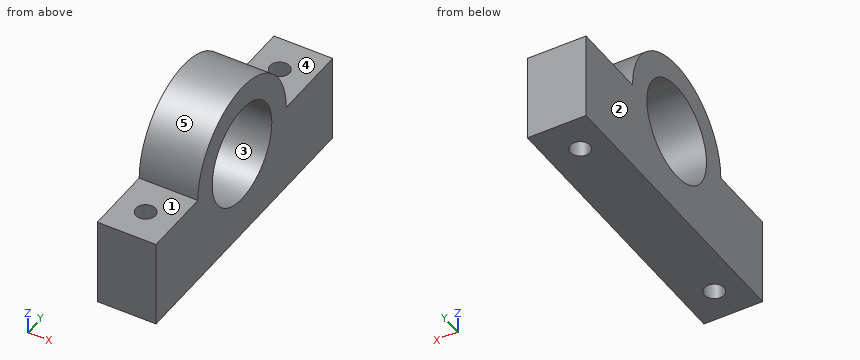
```python
from build123d import *

# Parameters (mm, degrees)
F1_DEPTH = 12.7
F2_R     = 2.1209
F3_DEPTH = 25.4
F4_R     = 2.1209
F5_DEPTH = 25.4


with BuildPart() as f1:
    # F0 (on Right) → F1 (new body)
    with BuildSketch(Plane.YZ):
        with BuildLine():
            Line((10.7188, 0), (15.875, 0))
            ThreePointArc((15.875, 0), (0, 15.875), (-15.875, 0))
            Line((-15.875, 0), (-10.7188, 0))
            ThreePointArc((-10.7188, 0), (0, 10.7188), (10.7188, 0))
        make_face()
        with BuildLine():
            Line((32.5907057375, 0), (15.875, 0))
            ThreePointArc((15.875, 0), (0, -15.875), (-15.875, 0))
            Line((-15.875, 0), (-30.9092942625, 0))
            Line((-30.9092942625, 0), (-30.9092942625, -19.05))
            Line((-30.9092942625, -19.05), (32.5907057375, -19.05))
            Line((32.5907057375, -19.05), (32.5907057375, 0))
        make_face()
        with BuildLine():
            ThreePointArc((-15.875, 0), (0, -15.875), (15.875, 0))
            Line((15.875, 0), (10.7188, 0))
            ThreePointArc((10.7188, 0), (0, -10.7188), (-10.7188, 0))
            Line((-10.7188, 0), (-15.875, 0))
        make_face()
    extrude(amount=F1_DEPTH)

    # F2 (on face) → F3 (cut)
    with BuildSketch(Plane.XY):
        with Locations((5.9564788826, 24.7918274254)):
            Circle(F2_R)
    extrude(amount=-F3_DEPTH, mode=Mode.SUBTRACT)

    # F4 (on face) → F5 (cut)
    with BuildSketch(Plane.XY):
        with Locations((6.1368788593, -23.7293746322)):
            Circle(F4_R)
    extrude(amount=-F5_DEPTH, mode=Mode.SUBTRACT)


solid = f1.part
```
Model file for the job. Use its own axes, mm. Face numbers are marked on the shaded views. A direction names the side the tool comes from. Coordinates: 2 decimals unless noted, no trailing zeros. Order: outer loops, then holes, each group sorted by start corner. A loop starts at its lowest first (then second) coordinate and runs counter-clockwise, first axis right, second up. Notation, with made-up numbers: (66, 54.5) -> (122, 54.5) arc R7 cw to (122, 63.5) -> close; hole circle Ø8 at (-37.75, 70). An arc over 180 degrees is marked (long way). Return JSON: item names as keys, results as strings.
Item 1: Slice it at D-D (x = 9.75). Write the cut outline in (y, z) (3 decimals), then the cut area to 3 significant figures.
Model answer:
{"outline": "(-30.909, -19.05) -> (32.591, -19.05) -> (32.591, 0) -> (15.875, 0) arc R15.875 ccw to (-15.875, 0) -> (-30.909, 0) -> close; hole circle Ø21.438 at (0, 0)", "area": "1,240 mm²"}
Item 2: Mould opens along Z. For the marked faces 1, 2 and 3 say: pulls with the +Z half, pulls with the -Z half, needs draft (parallel to the pull), parting line crosses it, or undercut.
Model answer:
{"face 1": "pulls with the +Z half", "face 2": "needs draft", "face 3": "undercut"}
Item 3: Slice it at A-A (y = 0). Write the cut outline in (x, z) (3 decimals).
Model answer:
{"outline": "(0, -19.05) -> (12.7, -19.05) -> (12.7, -10.719) -> (0, -10.719) -> close; (0, 10.719) -> (12.7, 10.719) -> (12.7, 15.875) -> (0, 15.875) -> close"}
Item 4: Slice it at B-B (z = -2). Write the cut outline in (x, y).
Model answer:
{"outline": "(0, -30.91) -> (12.7, -30.91) -> (12.7, -10.53) -> (0, -10.53) -> close; (0, 10.53) -> (12.7, 10.53) -> (12.7, 32.59) -> (0, 32.59) -> close; hole circle Ø4.24 at (5.96, 24.79); hole circle Ø4.24 at (6.14, -23.73)"}
Item 5: 3-axis set-ups, long thin cutter, end or side, ignore diameter. For the marked faces 4 and 5: which of +Z, -Z, +X, -X, +Y, -Y reach the whole face in a straight line?
Model answer:
{"face 4": "+Z, +X, -X, +Y", "face 5": "+Z, +X, -X"}
Item 6: Wall check: line 1 along Y through (x, z) = (7, -13.5); line 2 along Z through (x, y) = (7.75, 0) (3 decimals); line 3 along Y through (x, z) = (4.75, -3). Give the ranges that are in metal, low to high. Write a range as from..to.
Model answer:
{"line 1": "y = -30.91..-25.67, -21.79..22.95, 26.64..32.59", "line 2": "z = -19.05..-10.719, 10.719..15.875", "line 3": "y = -30.91..-25.33, -22.12..-10.29, 10.29..23.05, 26.54..32.59"}
Item 7: Pin check, flat tips, straight feed: P1, Ø5, axis at x = 6.14, y = -23.73, coming from the +Z side; P2, Ø5, axis at x = 3, z = 5, coming from the +Y side. Stop position of each tip, or through.
Model answer:
{"P1": "stops at z = 0", "P2": "stops at y = 15.68"}
Item 8: Slice it at C-C (x = 5.75). Write the cut outline in (y, z) (3 decimals).
Model answer:
{"outline": "(-30.909, -19.05) -> (-25.815, -19.05) -> (-25.815, 0) -> (-30.909, 0) -> close; (-21.644, -19.05) -> (22.681, -19.05) -> (22.681, 0) -> (15.875, 0) arc R15.875 ccw to (-15.875, 0) -> (-21.644, 0) -> close; (26.903, -19.05) -> (32.591, -19.05) -> (32.591, 0) -> (26.903, 0) -> close; hole circle Ø21.438 at (0, 0)"}
